Source: CAD feature listing. Evaluate the final solid. Frame: model axes, mm. A direction names the side the tool comes from. Coordinates: 2 decimals unless noted, no trailing zeros. Order: outer loops, then holes, each group sorted by start corner. A loop starts at its lowest first (then second) coordinate and runs counter-clockwise, first axis right, second up. Notation, with made-up numbers: (89, 76.25) -> (99, 76.25) arc R28 ccw to (99, 99.25) -> close; hole circle Ø11 at (51.25, 38). An arc over 180 degrees is marked (long way). Write item = value, one per line. Start each with the question number.
Item 1: Contact query for flat-ended pins moving along their axis: pin 1 (4.5 mm diameter, centred on y = 65, z = -6, fed in from -X); pin 2 (2 mm diameter, centred on y = 65, z = -36, fed in from -X); pin 3 (5 mm diameter, centred on x = 7, z = -64.5, fed in from -Y). Output: stop coordinate, or through.
Item 2: Ray query, line 1 along Y through (x, z) = (7.5, -36); line 2 along Z through (x, y) = (4.5, 47); line 3 along X through (y, z) = (22, -8.5). Return the intervals inside material, ascending. Write a range as [from, to].
Item 3: Set-up query: faces 1 (the flat face through (2.7, 38.38, -60.2)), 2 (the cylindrical face through (4.93, 0.554, -12.69)), 3 (the flat face through (4, 19.099, -31)). Return all of +Z, -Z, +X, -X, +Y, -Y with unobstructed straight access to the full face (end or side cutting, diameter ignored); none if empty.
Item 4: Section query A-A (z = -55). Output: boundary loops of the cut face in (x, y).
Item 5: Section query B-B (z = -114). Output: boundary loops of the cut face in (x, y).
Item 6: Section query C-C (y = 22). Count the separate pieces of the cut face and the enclosed holes in it, then the cut area to 3 significant figures.
Item 7: Mould query, pull axis Z, two halves, no side actions, for faces 4 (the flat face through (3, 70, -61)), 5 (the cylindrical face through (4.93, 0.9, -0.86)), 6 (the cylindrical face through (4.93, 66.15, -34.75)). Classes: released by +Z, released by -Z, zero draft, split by the parting line, or undercut.
```python
from build123d import *

# Parameters (mm, degrees)
SKETCH_1_R          = 1.7
EXTRUDE_1_DEPTH     = 10
CUT_EXTRUDE_1_DEPTH = 37
SKETCH_3_W          = 3
SKETCH_3_H          = 5.795399196
SKETCH_3_W_2        = 5.804634465
SKETCH_3_H_2        = 3.015219691
SKETCH_3_H_3        = 5.79316294
CUT_EXTRUDE_2_DEPTH = 8
SKETCH_5_R          = 1.7
CUT_EXTRUDE_3_DEPTH = 35
CUT_EXTRUDE_START   = -35
SKETCH_6_R          = 1.7
CUT_EXTRUDE_4_DEPTH = 35
CUT_EXTRUDE_5_DEPTH = 10
SKETCH_9_R          = 5
CUT_EXTRUDE_6_DEPTH = 10


with BuildPart() as part:
    # Эскиз1 → Бобышка-Вытянуть1 (new body)
    with BuildSketch(Plane(origin=(0, 0, 0), x_dir=(0, 0, -1), z_dir=(1, 0, 0))):
        with BuildLine():
            Line((3, 0), (10.95312335, 0))
            ThreePointArc((10.95312335, 0), (12.711116168, 0.569061652), (13.802171454, 2.060359164))
            Line((13.802171454, 2.060359164), (21.766885307, 26.20985548))
            Line((21.766885307, 26.20985548), (21.766885307, 27.126272908))
            ThreePointArc((21.766885307, 27.126272908), (11.12679914, 38.53238769), (26.145937625, 34.320931027))
            Line((26.145937625, 34.320931027), (26.145765698, 20.433139819))
            ThreePointArc((26.145765698, 20.433139819), (29.074654117, 13.361991979), (36.145765697, 10.433016021))
            Line((36.145765697, 10.433016021), (83.854234303, 10.433016021))
            ThreePointArc((83.854234303, 10.433016021), (90.925345883, 13.361991979), (93.854234302, 20.433139819))
            Line((93.854234302, 20.433139819), (93.854062375, 34.320931027))
            ThreePointArc((93.854062375, 34.320931027), (108.87320086, 38.53238769), (98.233114693, 27.126272908))
            Line((98.233114693, 27.126272908), (98.233114693, 26.20985548))
            Line((98.233114693, 26.20985548), (106.197828546, 2.060359164))
            ThreePointArc((106.197828546, 2.060359164), (107.288883832, 0.569061652), (109.04687665, 0))
            Line((109.04687665, 0), (117, 0))
            ThreePointArc((117, 0), (119.121320344, 0.878679656), (120, 3))
            Line((120, 3), (120, 67))
            ThreePointArc((120, 67), (119.121320344, 69.121320344), (117, 70))
            Line((117, 70), (3, 70))
            ThreePointArc((3, 70), (0.878679656, 69.121320344), (0, 67))
            Line((0, 67), (0, 3))
            ThreePointArc((0, 3), (0.878679656, 0.878679656), (3, 0))
        make_face()
        with Locations((36, 65)):
            Circle(SKETCH_1_R, mode=Mode.SUBTRACT)
        with Locations((6, 65)):
            Circle(SKETCH_1_R, mode=Mode.SUBTRACT)
        with Locations((36, 31)):
            Circle(SKETCH_1_R, mode=Mode.SUBTRACT)
        with Locations((84, 31)):
            Circle(SKETCH_1_R, mode=Mode.SUBTRACT)
        with Locations((84, 65)):
            Circle(SKETCH_1_R, mode=Mode.SUBTRACT)
        with Locations((114, 65)):
            Circle(SKETCH_1_R, mode=Mode.SUBTRACT)
        with BuildLine():
            Line((47, 65), (73, 65))
            ThreePointArc((73, 65), (75.121320344, 64.121320344), (76, 62))
            Line((76, 62), (76, 41.380344056))
            ThreePointArc((76, 41.380344056), (75.121320344, 39.259023712), (73, 38.380344056))
            Line((73, 38.380344056), (47, 38.380344056))
            ThreePointArc((47, 38.380344056), (44.878679656, 39.259023712), (44, 41.380344056))
            Line((44, 41.380344056), (44, 62))
            ThreePointArc((44, 62), (44.878679656, 64.121320344), (47, 65))
        make_face(mode=Mode.SUBTRACT)
        with BuildLine():
            Line((48.512942473, 28.14808317), (71.745561711, 28.14808317))
            ThreePointArc((71.745561711, 28.14808317), (76.161679417, 23.731965464), (71.745561711, 19.315847758))
            Line((71.745561711, 19.315847758), (48.512942473, 19.315847758))
            ThreePointArc((48.512942473, 19.315847758), (44.096824767, 23.731965464), (48.512942473, 28.14808317))
        make_face(mode=Mode.SUBTRACT)
    extrude(amount=EXTRUDE_1_DEPTH)

    # Эскиз2 → Вырез-Вытянуть1 (cut)
    with BuildSketch(Plane(origin=(0, 70, 0), x_dir=(1, 0, 0), z_dir=(0, 1, 0))):
        with BuildLine():
            ThreePointArc((7, 60), (6.414213562, 61.414213562), (5, 62))
            Line((5, 62), (5, 60))
            Line((5, 60), (7, 60))
        make_face()
        with BuildLine():
            Line((5, 60), (5, 62))
            ThreePointArc((5, 62), (3.585786438, 58.585786438), (7, 60))
            Line((7, 60), (5, 60))
        make_face()
    extrude(amount=-CUT_EXTRUDE_1_DEPTH, mode=Mode.SUBTRACT)

    # Эскиз3 → Вырез-Вытянуть2 (cut)
    with BuildSketch(Plane.ZY):
        with Locations((-89.477143784, 21.994873796)):
            Rectangle(SKETCH_3_W, SKETCH_3_H)
        with Locations((-60.018321185, 34.987499707)):
            Rectangle(SKETCH_3_W_2, SKETCH_3_H_2)
        with Locations((-30.522856216, 21.995572621)):
            Rectangle(SKETCH_3_W, SKETCH_3_H_3)
    extrude(amount=-CUT_EXTRUDE_2_DEPTH, mode=Mode.SUBTRACT)

    # Эскиз5 → Вырез-Вытянуть3 (cut)
    with BuildSketch(Plane(origin=(0, 0, -120), x_dir=(-1, 0, 0), z_dir=(0, 0, -1))):
        with Locations(Location((-5, 22, 0), (0, 0, 292.826701249))):
            Circle(SKETCH_5_R)
    extrude(amount=-CUT_EXTRUDE_3_DEPTH, mode=Mode.SUBTRACT)

    # Эскиз6 → Вырез-Вытянуть4 (cut)
    with BuildSketch(Plane.XY.offset(CUT_EXTRUDE_START)):
        with Locations(Location((5, 22, 0), (0, 0, 247.173298751))):
            Circle(SKETCH_6_R)
    extrude(amount=CUT_EXTRUDE_4_DEPTH, mode=Mode.SUBTRACT)

    # Эскиз7 → Вырез-Вытянуть5 (cut)
    with BuildSketch(Plane.ZY):
        Polygon((-76.161679417, 23.731965464), (-83.854234303, 10.433016021), (-36.145765697, 10.433016021), (-44.096824767, 23.731965464), align=None)
    extrude(amount=-CUT_EXTRUDE_5_DEPTH, mode=Mode.SUBTRACT)

    # Эскиз9 → Вырез-Вытянуть6 (cut)
    with BuildSketch(Plane.ZY):
        with Locations((-99.973969782, 53.749400687)):
            Circle(SKETCH_9_R)
        with Locations((-20.026030218, 53.749400687)):
            Circle(SKETCH_9_R)
    extrude(amount=-CUT_EXTRUDE_6_DEPTH, mode=Mode.SUBTRACT)


solid = part.part
```
Computed:
q1.pin_1 = 0
q1.pin_2 = through
q1.pin_3 = 28.15
q2.line_1 = [10.43, 29.3], [32.7, 63.3], [66.7, 70]
q2.line_2 = [-120, -76], [-44, 0]
q2.line_3 = [0, 3.3], [6.7, 10]
q3.face_1 = +X, -X
q3.face_2 = +X, -X, -Y
q3.face_3 = -X
q4.outline = (0, 28.15) -> (10, 28.15) -> (10, 38.38) -> (0, 38.38) -> close; (0, 65) -> (10, 65) -> (10, 70) -> (0, 70) -> close
q5.outline = (0, 0) -> (10, 0) -> (10, 63.3) -> (0, 63.3) -> close; (0, 66.7) -> (10, 66.7) -> (10, 70) -> (0, 70) -> close; hole circle Ø3.4 at (5, 22)
q6.separate_pieces = 8
q6.enclosed_holes = 0
q6.area = 517 mm^2
q7.face_4 = zero draft
q7.face_5 = released by +Z
q7.face_6 = undercut
